Could you check a few things on this model? Use its own coordinates, in mm. Face numbers are marked on the shaded views. A direction names the side the tool comes from. Give positions to 0.01 mm unless a question says otherwise; leave off trailing zeros. Loops run counter-clockwise (first coordinate to the right, second up) from the corner with the lowest first, then second, coordinate; pieces in that order, holes last. Notation, with made-up numbers: (-31.75, 79.5) - (-27.75, 79.5) arc R13 cw to (-27.75, 88.5) - close; hole circle Ø7 at (21, -10). An arc over 180 degrees is marked (long way). One line per item, written item: value. Start each with the question number.
Q1. I want a section at B-B (y = 21.3). Please give me the cut outline in (x, z).
Q2. I'm going to push flat-ended pins straight in: P1, Ø1, axis at x = 127, z = 15, coming from the +Y side; P2, Ø3, axis at x = 124.5, z = 15.5, coming from the +Y side. Where does each tip first touch, or does it pass through?
Q3. I want a section at A-A (x = 125.3). Please give me the cut outline in (y, z).
Q4. If I drill on line 1 (Y direction, x = 125.35, z = 27.25); line 2 (Y direction, x = 124.75, z = 26.75); line 3 (X direction, y = 23.3, z = 26.5), over which ranges is the centre line in solid material (lowest first)? Write a range as from..to.
Q5. I want a section at C-C (z = 22.75). Please give me the cut outline in (x, y).
Q6. For the marked faces 1, 2 and 3, which set-ups out of +Z, -Z, +X, -X, +Y, -Y let a thin tool reach every point of the face, with its end or its side?
```python
from build123d import *

# Parameters (mm, degrees)
SKETCH040_R       = 2.2
PAD032_DEPTH      = 17.3
CYLINDER002_R     = 2.6
CYLINDER002_DEPTH = 1
FILLET005_R       = 0.25


with BuildPart() as part:
    # Sketch040 → Pad032 (new body)
    with BuildSketch(Plane.XY):
        with Locations((125.3, 21.3)):
            Circle(SKETCH040_R)
    extrude(amount=PAD032_DEPTH)

    # Cylinder002 → Cylinder002 (join)
    with BuildSketch(Plane(origin=(125.3, 21.3, 13.3), x_dir=(1, 0, 0), z_dir=(0, 0, 1))):
        Circle(CYLINDER002_R)
    extrude(amount=CYLINDER002_DEPTH)

    # Fillet005
    fillet005_edges = [part.edges().sort_by_distance(p)[0] for p in [
        (122.7, 21.3, 14.3),
        (122.7, 21.3, 13.3),
        (123.1, 21.3, 17.3),
        (123.1, 21.3, 0),
    ]]
    fillet(fillet005_edges, radius=FILLET005_R)


with BuildPart() as part_1:
    # Body034 placement: moved
    add(part.part.moved(Location((0, 0, 12))))


solid = part_1.part
```
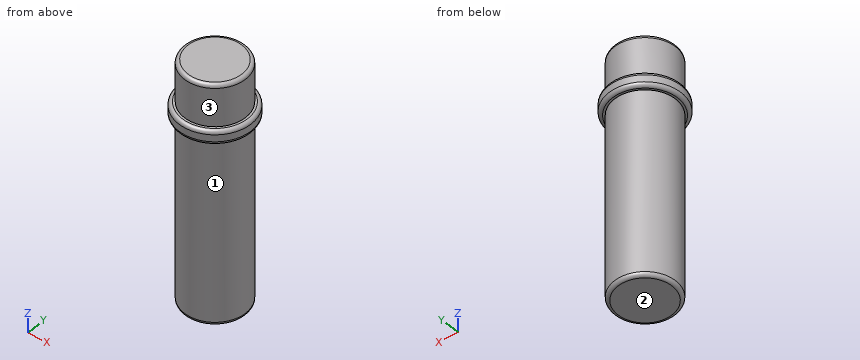
Worked answers:
1. outline: (122.7, 25.55) arc R0.25 ccw to (122.95, 25.3) - (123.1, 25.3) - (123.1, 12.25) arc R0.25 ccw to (123.35, 12) - (127.25, 12) arc R0.25 ccw to (127.5, 12.25) - (127.5, 25.3) - (127.65, 25.3) arc R0.25 ccw to (127.9, 25.55) - (127.9, 26.05) arc R0.25 ccw to (127.65, 26.3) - (127.5, 26.3) - (127.5, 29.05) arc R0.25 ccw to (127.25, 29.3) - (123.35, 29.3) arc R0.25 ccw to (123.1, 29.05) - (123.1, 26.3) - (122.95, 26.3) arc R0.25 ccw to (122.7, 26.05) - close
2. P1: stops at y = 23.14
2. P2: stops at y = 23.5
3. outline: (18.7, 25.55) arc R0.25 ccw to (18.95, 25.3) - (19.1, 25.3) - (19.1, 12.25) arc R0.25 ccw to (19.35, 12) - (23.25, 12) arc R0.25 ccw to (23.5, 12.25) - (23.5, 25.3) - (23.65, 25.3) arc R0.25 ccw to (23.9, 25.55) - (23.9, 26.05) arc R0.25 ccw to (23.65, 26.3) - (23.5, 26.3) - (23.5, 29.05) arc R0.25 ccw to (23.25, 29.3) - (19.35, 29.3) arc R0.25 ccw to (19.1, 29.05) - (19.1, 26.3) - (18.95, 26.3) arc R0.25 ccw to (18.7, 26.05) - close
4. line 1: y = 19.1..23.5
4. line 2: y = 19.17..23.43
4. line 3: x = 124.38..126.22
5. outline: circle Ø4.4 at (125.3, 21.3)
6. face 1: -Z
6. face 2: -Z, +X, -X, +Y, -Y
6. face 3: +Z
